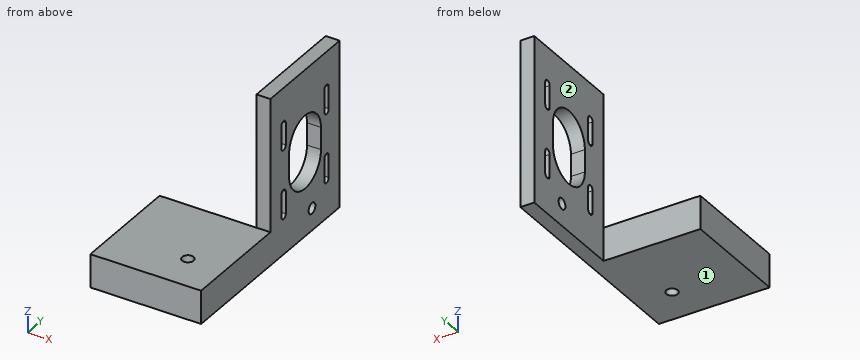
from build123d import *

# Parameters (mm, degrees)
SKETCH_W        = 50
SKETCH_H        = 50
PAD_DEPTH       = 15
SKETCH001_W     = 6.3
SKETCH001_H     = 50
PAD001_DEPTH    = 75
SKETCH002_R     = 2.45
POCKET_DEPTH    = 13
SKETCH004_R     = 2.6
POCKET001_DEPTH = 85.001


with BuildPart() as part:
    # Sketch → Pad (new body)
    with BuildSketch(Plane.XY):
        with Locations((-25, -25)):
            Rectangle(SKETCH_W, SKETCH_H)
    extrude(amount=PAD_DEPTH)

    # Sketch001 → Pad001 (join)
    with BuildSketch(Plane.XY):
        with Locations((-3.15, 25)):
            Rectangle(SKETCH001_W, SKETCH001_H)
    extrude(amount=PAD001_DEPTH)

    # Sketch002 (on Face12 of Pad001) → Pocket (cut)
    with BuildSketch(Plane.YZ):
        with Locations((30, 10)):
            Circle(SKETCH002_R)
        with BuildLine():
            ThreePointArc((42.1, 58.5), (40.5, 60.1), (38.9, 58.5))
            Line((38.9, 58.5), (38.9, 48.5))
            ThreePointArc((38.9, 48.5), (40.5, 46.9), (42.1, 48.5))
            Line((42.1, 58.5), (42.1, 48.5))
        make_face()
        with BuildLine():
            ThreePointArc((42.1, 27.5), (40.5, 29.1), (38.9, 27.5))
            Line((38.9, 27.5), (38.9, 17.5))
            ThreePointArc((38.9, 17.5), (40.5, 15.9), (42.1, 17.5))
            Line((42.1, 27.5), (42.1, 17.5))
        make_face()
        with BuildLine():
            ThreePointArc((11.1, 58.5), (9.5, 60.1), (7.9, 58.5))
            Line((7.9, 58.5), (7.9, 48.5))
            ThreePointArc((7.9, 48.5), (9.5, 46.9), (11.1, 48.5))
            Line((11.1, 58.5), (11.1, 48.5))
        make_face()
        with BuildLine():
            ThreePointArc((11.1, 27.5), (9.5, 29.1), (7.9, 27.5))
            Line((7.9, 27.5), (7.9, 17.5))
            ThreePointArc((7.9, 17.5), (9.5, 15.9), (11.1, 17.5))
            Line((11.1, 27.5), (11.1, 17.5))
        make_face()
        with BuildLine():
            ThreePointArc((36.5, 43), (25, 54.5), (13.5, 43))
            Line((13.5, 43), (13.5, 33))
            ThreePointArc((13.5, 33), (25, 21.5), (36.5, 33))
            Line((36.5, 43), (36.5, 33))
        make_face()
    extrude(amount=-POCKET_DEPTH, mode=Mode.SUBTRACT)

    # Sketch004 → Pocket001 (cut, through all)
    with BuildSketch(Plane(origin=(0, 0, -10), x_dir=(1, 0, 0), z_dir=(0, 0, -1))):
        with Locations((-16.55, 33.05)):
            Circle(SKETCH004_R)
    extrude(amount=-POCKET001_DEPTH, mode=Mode.SUBTRACT)


solid = part.part
Design review of the part built by this model. Coordinates are the model's own, in mm. Face numbers are marked on the shaded views. A direction names the side the tool comes from. Give positions to 0.01 mm unless a question says otherwise; leave off trailing zeros. Write each loop counter-clockwise with the first axis right and the second up, starting at its lowest first coordinate (ties: lowest second). Pieces come first, ordered by that corner, then holes. Notation, with made-up numbers: M 31,-32.5 L 85,-32.5 A24 ccw 85,-14.5 Z; hole C 85.5,73 d5. An arc over 180 degrees is marked long. Answer as a JSON object with one key per item and string values. Group by question number.
1) For line 1 along X through (y, z) = (-33.05, 11.75); line 2 along Z through (x, y) = (-3, 30); line 3 along X through (y, z) = (32, 23.5), list the stretches that pass through material, from the lowest coordinate up.
2) Clearance check with flat-ended pins moving along their axes: pin 1 Ø1 at (x, y) = (-13, 0) entering from +Z; pin 2 Ø8 at (y, z) = (30, 10) entering from -X; pin 3 Ø3 at (x, z) = (-4, 24.5) entering from -Y. State where each tip first meets the part, or that it passes through.
3) We need section A-A (z = 10). Give the boundary of the cut face in (x, y), and give its area (3 significant figures).
4) Tool access review of the marked faces 1 and 2: name each direction out of +Z, -Z, +X, -X, +Y, -Y from which nothing blocks a thin tool from reaching the whole face with its end or side.
5) We need section C-C (x = -16.55). Give the boundary of the cut face in (y, z), and give its area (3 significant figures).
6) We need section D-D (y = -33.05). Give the boundary of the cut face in (x, z).
7) We need section B-B (y = 9.5). Give the boundary of the cut face in (x, z).
Answer key:
{
 "1": {"line 1": "x = -50 to -19.15, -13.95 to 0", "line 2": "z = 0 to 7.55, 12.45 to 22.64, 53.36 to 75", "line 3": "x = -6.3 to 0"},
 "2": {"pin 1": "stops at z = 15", "pin 2": "stops at x = -6.3", "pin 3": "stops at y = 0"},
 "3": {"outline": "M -50,-50 L 0,-50 L 0,27.55 L -6.3,27.55 L -6.3,0 L -50,0 Z; M -6.3,32.45 L 0,32.45 L 0,50 L -6.3,50 Z; hole C -16.55,-33.05 d5.2", "area": "2,760 mm²"},
 "4": {"face 1": "-Z, +X, -X, +Y, -Y", "face 2": "+Z, -Z, -X, +Y"},
 "5": {"outline": "M -50,0 L -35.65,0 L -35.65,15 L -50,15 Z; M -30.45,0 L 0,0 L 0,15 L -30.45,15 Z", "area": "672 mm²"},
 "6": {"outline": "M -50,0 L -19.15,0 L -19.15,15 L -50,15 Z; M -13.95,0 L 0,0 L 0,15 L -13.95,15 Z"},
 "7": {"outline": "M -6.3,0 L 0,0 L 0,15.9 L -6.3,15.9 Z; M -6.3,29.1 L 0,29.1 L 0,46.9 L -6.3,46.9 Z; M -6.3,60.1 L 0,60.1 L 0,75 L -6.3,75 Z"}
}
